Input: part model. Units: mm. Frame: model coordinates. A direction names the side the tool comes from. Round coordinates to 2 decimals unless told otherwise and drop trailing zeros. Loops run counter-clockwise (first coordinate to the right, second up) from the corner with the lowest first, then second, coordinate; pieces in that order, holes last. Notation, with made-up numbers: (-19, 11) -> (-10, 11) arc R23 cw to (-10, 30) -> close; hole circle Ø10 at (-18, -13.5). An arc over 180 degrees is marked (long way). One line per question, with ' | ' between items. Start each with the question number.
Q1. Cut plane B-B on z = 0. Return loops of the section in (x, y), and give its area (3 significant figures).
Q2. Cut plane A-A on x = 0. Return loops of the section in (y, z), and give its area (3 significant figures).
Q3. Mould query, pull axis X, two halves, no side actions, for faces 1 (the face through (-7.1, -15.68, 5.45)), 2 (the face through (-9.632, 2.268, -12.812)), 3 (the face through (0, 4.6, -4)), 4 (the face through (-2.8, 2.33, -24.57)). Classes: pulls with the +X half, pulls with the -X half, needs draft (parallel to the pull), parting line crosses it, or undercut.
Q4. Cut plane C-C on z = -22. Return loops of the section in (x, y), and give its area (3 significant figures).
Q5. Contact query for flat-ended pins moving along their axis: P1, Ø3, axis at y = -23, z = 4, coming from the +X side; P2, Ø4, axis at x = 6, y = -23, coming from the +Z side; P3, Ø5, axis at x = -1, y = -5.5, coming from the -Z side. Output: stop coordinate, or through.
Q6. Access query for faces 5 (the face through (0.2, 0, -9.1)), 6 (the face through (-0.1, 2.3, -29.6)). Directions: +Z, -Z, +X, -X, +Y, -Y. A direction counts if a zero-diameter tool reaches every point of the face in a straight line with its end or side. Return the directions, or none.
Q7. Material intervals for L1, parallel to Z at x = 0, y = 2.4; L2, parallel to Y at x = 7.25, z = -8; L3, parallel to X at y = 3, z = -22, sorted ascending.
Q8. Cut plane D-D on y = -6. Return loops of the section in (x, z), and give its area (3 significant figures).
from build123d import *

# Parameters (mm, degrees)
BASE_DEPTH               = 4.6
SKETCH4_R                = 8.95
SENSOR_DEPTH             = 31.8
BOLT_HOLE_M7_CLEARANCE_D = 7.6


with BuildPart() as part:
    # Sketch1 → Base (new body)
    with BuildSketch(Plane(origin=(0, 0, 0), x_dir=(1, 0, 0), z_dir=(0, 1, 0))):
        with BuildLine():
            Line((-11.757550765, 2.4), (-7.446448818, 23.52))
            ThreePointArc((-7.446448818, 23.52), (0, 29.6), (7.446448818, 23.52))
            Line((7.446448818, 23.52), (11.757550765, 2.4))
            ThreePointArc((11.757550765, 2.4), (0, -12), (-11.757550765, 2.4))
        make_face()
    extrude(amount=BASE_DEPTH)

    # Sketch4 → Sensor (add)
    with BuildSketch(Plane(origin=(0, 0, 0), x_dir=(1, 0, 0), z_dir=(0, 1, 0))):
        Circle(SKETCH4_R)
    extrude(amount=-SENSOR_DEPTH)

    # Bolt Hole (M7 Clearance) (through all)
    with Locations(Plane(origin=(0, 0, 0), x_dir=(-1, 0, 0), z_dir=(0, -1, 0))):
        with Locations((0, 22)):
            Hole(BOLT_HOLE_M7_CLEARANCE_D / 2)


solid = part.part
Results:
1) outline: (-12, 0) -> (-8.95, 0) -> (-8.95, -31.8) -> (8.95, -31.8) -> (8.95, 0) -> (12, 0) -> (12, 4.6) -> (-12, 4.6) -> close | area: 680 mm^2
2) outline: (-31.8, -8.95) -> (0, -8.95) -> (0, -18.2) -> (4.6, -18.2) -> (4.6, 12) -> (0, 12) -> (0, 8.95) -> (-31.8, 8.95) -> close; (0, -29.6) -> (4.6, -29.6) -> (4.6, -25.8) -> (0, -25.8) -> close | area: 726 mm^2
3) face 1: parting line crosses it | face 2: pulls with the -X half | face 3: needs draft | face 4: undercut
4) outline: (-7.76, 0) -> (-3.8, 0) -> (-3.8, 4.6) -> (-7.76, 4.6) -> close; (3.8, 0) -> (7.76, 0) -> (7.76, 4.6) -> (3.8, 4.6) -> close | area: 36.4 mm^2
5) P1: x = 8.59 | P2: z = 8.01 | P3: z = -8.95
6) face 5: -Y | face 6: -Z, +Y, -Y
7) L1: -29.6 to -25.8, -18.2 to 12 | L2: 0 to 4.6 | L3: -7.76 to -3.8, 3.8 to 7.76
8) outline: circle Ø17.9 at (0, 0) | area: 252 mm^2
